```python
from build123d import *

# Parameters (mm, degrees)
F0_W        = 38.1
F0_H        = 914.4
F0_R        = 6.35
F1_DEPTH    = 139.7
F2_R        = 6.35
F3_DEPTH    = 38.1
F6_R        = 6.35
F7_DEPTH    = 38.1
F8_D        = 6.35
F4_R        = 12.7
F5_R        = 6.35
F9_T1_DEPTH = 139.7
F9_T4_ANGLE = 90
F9_T6_ANGLE = 90


# Not quite as in the source:
# - a fillet or chamfer that OpenCascade refuses, or shapes differently, is made with other operations: its cross-section is extruded or revolved along the edge and cut away or added


with BuildPart() as f1:
    # F0 (on Front) → F1 (new body)
    with BuildSketch(Plane.XZ):
        Rectangle(F0_W, F0_H)
        with Locations((0, 398.018)):
            Circle(F0_R, mode=Mode.SUBTRACT)
        with Locations((0, 427.482)):
            Circle(F0_R, mode=Mode.SUBTRACT)
    extrude(amount=-F1_DEPTH)

    # F2 (on face) → F3 (cut)
    with BuildSketch(Plane(origin=(-19.05, 0, 0), x_dir=(0, -1, 0), z_dir=(-1, 0, 0))):
        with Locations((-93.1418, -427.482)):
            Circle(F2_R)
        with Locations((-93.1418, -398.018)):
            Circle(F2_R)
        with Locations((-46.5836, -427.482)):
            Circle(F2_R)
        with Locations((-46.5836, -398.018)):
            Circle(F2_R)
    extrude(amount=-F3_DEPTH, mode=Mode.SUBTRACT)

    # F6 (on face) → F7 (cut)
    with BuildSketch(Plane(origin=(-19.05, 0, 0), x_dir=(0, -1, 0), z_dir=(-1, 0, 0))):
        with Locations((-69.85, -21.336)):
            Circle(F6_R)
        with Locations((-69.85, -50.8)):
            Circle(F6_R)
    extrude(amount=-F7_DEPTH, mode=Mode.SUBTRACT)

    # F8 (through all)
    with Locations(Plane(origin=(-19.05, 0, 0), x_dir=(0, -1, 0), z_dir=(-1, 0, 0))):
        with Locations((-107.95, 283.21), (-107.95, 190.246), (-107.95, 97.282)):
            Hole(F8_D / 2)

    # F4
    f4_edges = [f1.edges().sort_by_distance(p)[0] for p in [
        (19.05, 69.85, 457.2),
        (-19.05, 69.85, -457.2),
        (19.05, 69.85, -457.2),
    ]]
    fillet(f4_edges, radius=F4_R)

    # F5
    f5_edges = [f1.edges().sort_by_distance(p)[0] for p in [
        (-19.05, 0, 6.35),
        (19.05, 0, 0),
        (19.05, 139.7, 0),
    ]]
    fillet(f5_edges, radius=F5_R)

    # F9: fillet of radius 25.4 on 1 edges, made by hand

    # F9_s2 → F9_t1 (cut)
    with BuildSketch(Plane.XZ.offset(-139.7)):
        with BuildLine():
            ThreePointArc((6.35, 457.2), (-11.6105122421, 449.7605122421), (-19.05, 431.8))
            Line((-19.05, 431.8), (-19.05, 457.2))
            Line((-19.05, 457.2), (6.35, 457.2))
        make_face()
    extrude(amount=F9_T1_DEPTH, mode=Mode.SUBTRACT)

    # F9_s3 → F9_t4 (revolve, cut)
    with BuildSketch(Plane.YZ.offset(6.35)):
        with BuildLine():
            ThreePointArc((0, 450.85), (1.8598719395, 455.3401280605), (6.35, 457.2))
            Line((6.35, 457.2), (0, 457.2))
            Line((0, 457.2), (0, 450.85))
        make_face()
    revolve(axis=Axis((6.35, 0, 431.8), (0, -1, 0)), revolution_arc=F9_T4_ANGLE, mode=Mode.SUBTRACT)

    # F9_s5 → F9_t6 (revolve, cut)
    with BuildSketch(Plane.XY.offset(431.8)):
        with BuildLine():
            ThreePointArc((-12.7, 139.7), (-17.1901280605, 137.8401280605), (-19.05, 133.35))
            Line((-19.05, 133.35), (-19.05, 139.7))
            Line((-19.05, 139.7), (-12.7, 139.7))
        make_face()
    revolve(axis=Axis((6.35, 139.7, 431.8), (0, 1, 0)), revolution_arc=F9_T6_ANGLE, mode=Mode.SUBTRACT)


solid = f1.part
```
Build history of the part. All positions in model axes, mm. Give positions to 0.01 mm unless a question says otherwise; leave off trailing zeros.
1) Two-plate mould, pull along X, no slides. Class faces 1 (the face through (-19.05, 69, -12)), 2 (the face through (19.05, 69, -6)), 3 (the face through (0, 139.7, 6)): released by +X, released by -X, zero draft, split by the parting line, or undercut.
Values follow:
face 1: released by -X
face 2: released by +X
face 3: zero draft
2) Band-saw the part on A-A on x = 0. State how many separate pieces and enclosed holes the cut face has, then the cut area to 3 significant figures.
Values follow:
separate pieces: 3
enclosed holes: 9
area: 123,000 mm2
3) Probe line 1 along Z through (x, y) = (7.5, 69.85); line 2 along Z through (x, y) = (0, 74.5); line 3 along Z through (x, y) = (-12.5, 105.5). List the from-to ranges inside material, lowest first.
Values follow:
line 1: z = -457.15 to -57.15, -44.45 to -27.69, -14.99 to 457.15
line 2: z = -457.2 to -55.12, -46.48 to -25.66, -17.01 to 391.67, 404.37 to 421.13, 433.83 to 456.39
line 3: z = -455.61 to 95.26, 99.3 to 188.23, 192.27 to 281.19, 285.23 to 448.82
4) Drop flat-ended pins along their axis: P1, Ø12, axis at x = -2.5, y = 98, coming from the +Z side; P2, Ø6, axis at x = -13, y = 41, coming from the -Z side. Give the stop position or say it passes through.
Values follow:
P1: stops at z = 457.04
P2: stops at z = -456.66
